from build123d import *

# Parameters (mm, degrees)
SKETCH_W     = 5.2
SKETCH_H     = 5.2
PAD_DEPTH    = 40
SKETCH001_R  = 5
PAD001_DEPTH = 27
POCKET_DEPTH = 22


with BuildPart() as part:
    # Sketch → Pad (new body)
    with BuildSketch(Plane.XY):
        Rectangle(SKETCH_W, SKETCH_H)
    extrude(amount=PAD_DEPTH)

    # Sketch001 → Pad001 (new body)
    with BuildSketch(Plane.XY.offset(40)):
        Circle(SKETCH001_R)
    extrude(amount=PAD001_DEPTH)

    # Sketch002 → Pocket (cut)
    with BuildSketch(Plane.XY.offset(67)):
        with BuildLine():
            Line((-1.697056, 2.1), (1.697056, 2.1))
            ThreePointArc((-1.697056, 2.1), (0, -2.7), (1.697056, 2.1))
        make_face()
    extrude(amount=-POCKET_DEPTH, mode=Mode.SUBTRACT)


solid = part.part
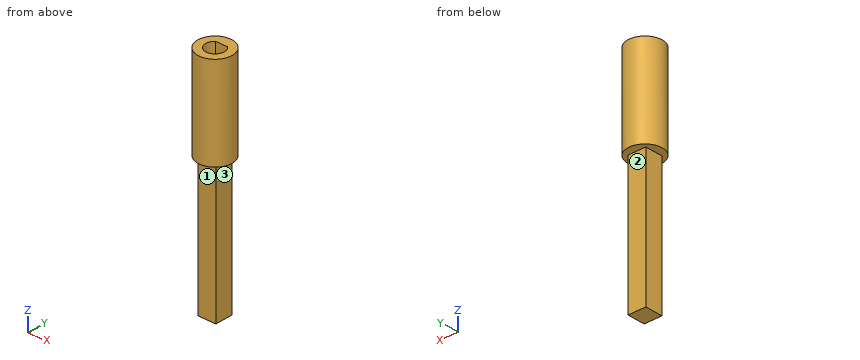
Build history of the part. All positions in model axes, mm. Face numbers are marked on the shaded views. A direction names the side the tool comes from. Give positions to 0.01 mm unless a question says otherwise; leave off trailing zeros. Order: outer loops, then holes, each group sorted by start corner. A loop starts at its lowest first (then second) coordinate and runs counter-clockwise, first axis right, second up. Notation, with made-up numbers: M 87.5,8 L 137.5,8 A17 cw 137.5,40 Z; hole C 38.25,53 d1. An arc over 180 degrees is marked long. Use one line per item in the form item = value.
Q1. Slice it at C-C, the plane z = 60. Write the cut outline in (x, y), and give its area (3 significant figures).
Conclusion:
outline = C 0,0 d10; hole M -1.7,2.1 A2.7 ccw long 1.7,2.1 Z
area = 57.0 mm2
Q2. Wall check: probe 1 along Y at (x, z) = (0, 62.25); probe 2 along Z at (x, y) = (-0.5, 0.5); probe 3 along X at (y, z) = (1.5, 12). Give the ranges that are in metal, low to high.
Conclusion:
probe_1 = -5 to -2.7, 2.1 to 5
probe_2 = 0 to 45
probe_3 = -2.6 to 2.6
Q3. Pin check, flat tips, straight feed: P1, Ø2, axis at y = -3.5, z = 37.5, coming from the +X side; P2, Ø2, axis at x = -3.5, z = 40, coming from the +Y side; P3, Ø3, axis at x = -0.5, y = -3, coming from the -Z side; P4, Ø4, axis at x = 1, z = 20, coming from the +Y side. Stop position of each tip, or through.
Conclusion:
P1 = 2.6
P2 = 4.33
P3 = 0
P4 = 2.6
Q4. Slice it at A-A, the plane y = 0. Write the cut outline in (x, z).
Conclusion:
outline = M -5,40 L -2.6,40 L -2.6,0 L 2.6,0 L 2.6,40 L 5,40 L 5,67 L 2.7,67 L 2.7,45 L -2.7,45 L -2.7,67 L -5,67 Z
Q5. Which spindle directions (+Z, -Z, +X, -X, +Y, -Y) get a long thin tool onto all of the face, cutting with end or side? Do the marked faces 1, 2 and 3. Say none if no direction does.
Conclusion:
face_1 = -Z, +X, -X, -Y
face_2 = -Z, +X, -X, +Y
face_3 = -Z, +X, +Y, -Y
Q6. Slice it at B-B, the plane x = 0. Write the cut outline in (y, z), and give its area (3 significant figures).
Conclusion:
outline = M -5,40 L -2.6,40 L -2.6,0 L 2.6,0 L 2.6,40 L 5,40 L 5,67 L 2.1,67 L 2.1,45 L -2.7,45 L -2.7,67 L -5,67 Z
area = 372 mm2
Q7. Slice it at D-D, the plane z = 43.5. Write the cut outline in (x, y), and give its area (3 significant figures).
Conclusion:
outline = C 0,0 d10
area = 78.5 mm2
